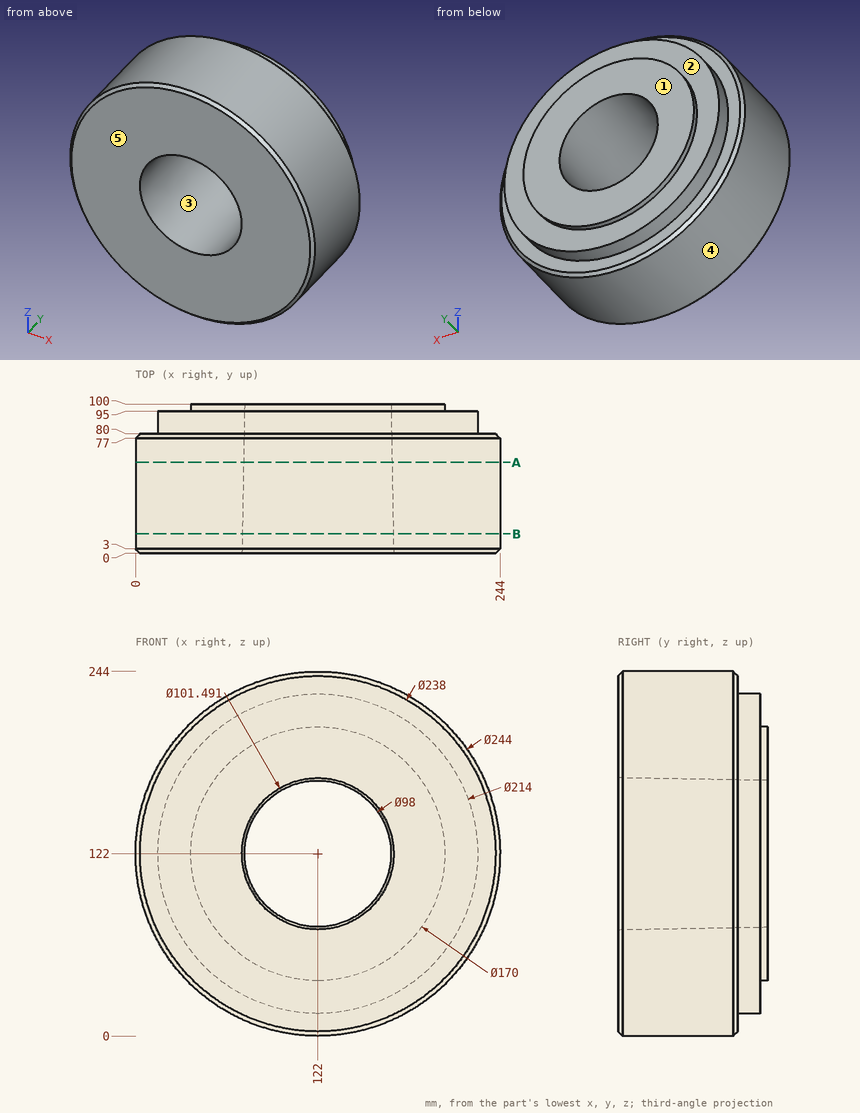
Design review of the part shown in the three views and the two pictorial views. Dimensions are in mm from the part's minimum x, y and z. A direction names the side the tool comes from. Coordinates: 2 decimals unless noted, no trailing zeros. Loops run counter-clockwise (first coordinate to the right, second up) from the corner with the lowest first, then second, coordinate; pieces in that order, holes last. Notation, with made-up numbers: (64, 55.5) - (82, 55.5) arc R27 ccw to (82, 75.5) - close; hole circle Ø11 at (49.25, 88). An arc over 180 degrees is marked (long way). Use a Markdown table: item, result. Add a question column.
Item 1: For line 1 (Y direction, x = 37.5, z = 62.5); line 2 (Y direction, x = 194, z = 30.5); line 3 (Z direction, x = 77, y = 54), list the stretches that pass through material, from the lowest coordinate up.
Item 2: Tool access review of the marked faces 1 and 2: name each direction out of +Z, -Z, +X, -X, +Y, -Y from which nothing blocks a thin tool from reaching the whole face with its end or side.
Item 3: We need section B-B (y = 13). Give the boundary of the cut face in (x, z), and give its area (3 significant figures).
Item 4: Mouldability with a two-part tool opening along X and no side actions: class the marked faces 3, 4 and 5 as pulls with the +X half, pulls with the -X half, needs draft (parallel to the pull), parting line crosses it, or undercut.
Item 5: Insertion check: pin 1 Ø3 at (y, z) = (84, 199) entering from -X; pin 2 Ø12 at (x, y) = (46, 23.5) entering from -Z; pin 3 Ø4 at (x, y) = (139, 81.5) entering from +Z. Each pin has a flat end and moves straight along its axis. Give the tip position at first contact, or say it passes through.
Item 6: We need section A-A (y = 61). Give the boundary of the cut face in (x, z), and give its area (3 significant figures).
Results list:
| question | item | result |
|---|---|---|
| 1 | line 1 | y = 0 to 95 |
| 1 | line 2 | y = 0 to 80 |
| 1 | line 3 | z = 8.6 to 100.66, 143.34 to 235.4 |
| 2 | face 1 | +Z, -Z, +X, -X, +Y |
| 2 | face 2 | +Y |
| 3 | outline | circle Ø244 at (122, 122); hole circle Ø101.04 at (122, 122) |
| 3 | area | 38,700 mm^2 |
| 4 | face 3 | undercut |
| 4 | face 4 | parting line crosses it |
| 4 | face 5 | needs draft |
| 5 | pin 1 | stops at x = 46.18 |
| 5 | pin 2 | stops at z = 22.08 |
| 5 | pin 3 | stops at z = 240.3 |
| 6 | outline | circle Ø244 at (122, 122); hole circle Ø99.36 at (122, 122) |
| 6 | area | 39,000 mm^2 |
